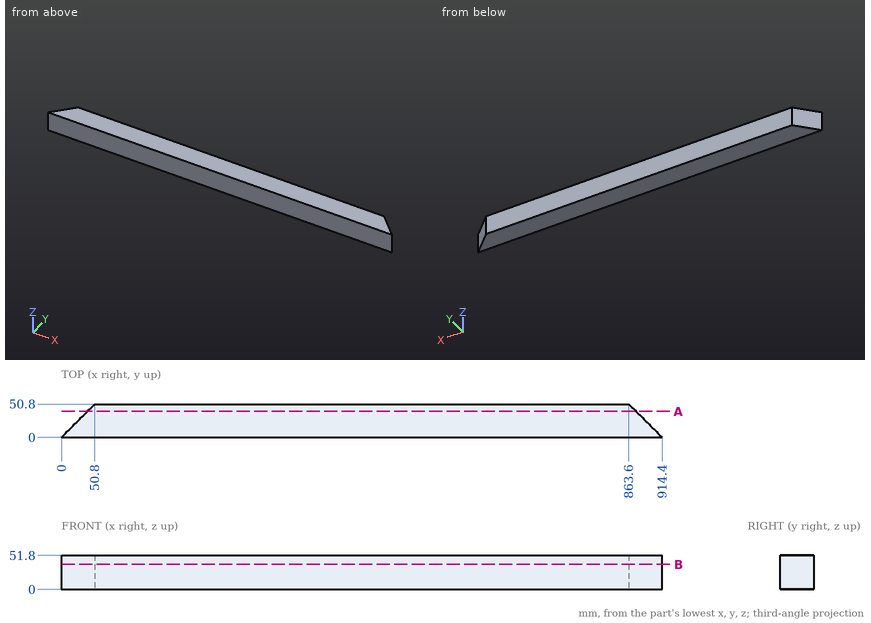
Print and shaded views of the part. All mm, measured from the part's lowest x, y and z. Give positions to 0.01 mm unless a question says otherwise; leave off trailing zeros. Write each loop counter-clockwise with the first axis right and the second up, starting at its lowest first coordinate (ties: lowest second). Pieces come first, ordered by that corner, then holes. Notation, with made-up numbers: (42, -2.75) - (85, -2.75) arc R14 ccw to (85, 5.25) - close; hole circle Ø1 at (89.25, 48). An arc over 180 degrees is marked (long way). One line per question, with ' | ' between items. Start each with the question number.
(1) Slice it at B-B on z = 38. Write the cut outline in (x, y), plus the area to 3 significant figures.
(2) Wall check: line 1 along X through (y, z) = (18.5, 43); line 2 along X through (y, z) = (4.5, 40.5); line 3 along Y through (x, z) = (47, 14). Give the ranges that are in metal, low to high. Write a range as from..to.
(3) Pin check, flat tips, straight feed: P1, Ø6, axis at y = 29, z = 30.5, coming from the -X side; P2, Ø12, axis at y = 26, z = 37, coming from the +X side; P3, Ø5, axis at y = 8.5, z = 17, coming from the +X side. Stop position of each tip, or through.
(4) Slice it at A-A on y = 39.5. Write the cut outline in (x, z), plus the area to 3 significant figures.
Results below:
1) outline: (0, 0) - (914.4, 0) - (863.6, 50.8) - (50.8, 50.8) - close | area: 43,900 mm^2
2) line 1: 18.5..895.9 | line 2: 4.5..909.9 | line 3: 0..47
3) P1: x = 26 | P2: x = 894.4 | P3: x = 908.4
4) outline: (39.5, 0) - (874.9, 0) - (874.9, 51.8) - (39.5, 51.8) - close | area: 43,300 mm^2
